Can you work these out from the drawing? Everything is in mm from the part's minimum corner. Coordinates: 2 decimals unless noted, no trailing zeros. Order: outer loops, then holes, each group sorted by start corner. A loop starts at its lowest first (then second) coordinate and runs counter-clockwise, first axis right, second up. Notation, with made-up numbers: (43, -31) -> (101, -31) arc R16 cw to (101, -5) -> close; hole circle Ø3 at (63.25, 82.5). An arc over 180 degrees is marked (long way). Return JSON: item names as keys, results as strings. Group by question number.
1) If I drill on probe 1 along Y at (x, z) = (93, 0.85); probe 2 along Y at (x, z) = (5, 0.9); probe 3 along X at (y, z) = (60, 1.85), over which ranges is the centre line in solid material (lowest first)? Write a range as from..to.
2) If we section it at B-B, the plane x = 35: Please give me the cut outline in (y, z), then the cut area to 3 significant figures.
3) For pin 1 (1.5 mm diameter, centred on x = 93, y = 59, fed in from +Z), with a flat end and sliding along its axis, tell me the tip position at first contact or that it passes through.
4) If we section it at A-A, the plane y = 10: Please give me the cut outline in (x, z), then the cut area to 3 significant figures.
5) If we section it at C-C, the plane x = 5: Please give me the cut outline in (y, z), then the cut area to 3 significant figures.
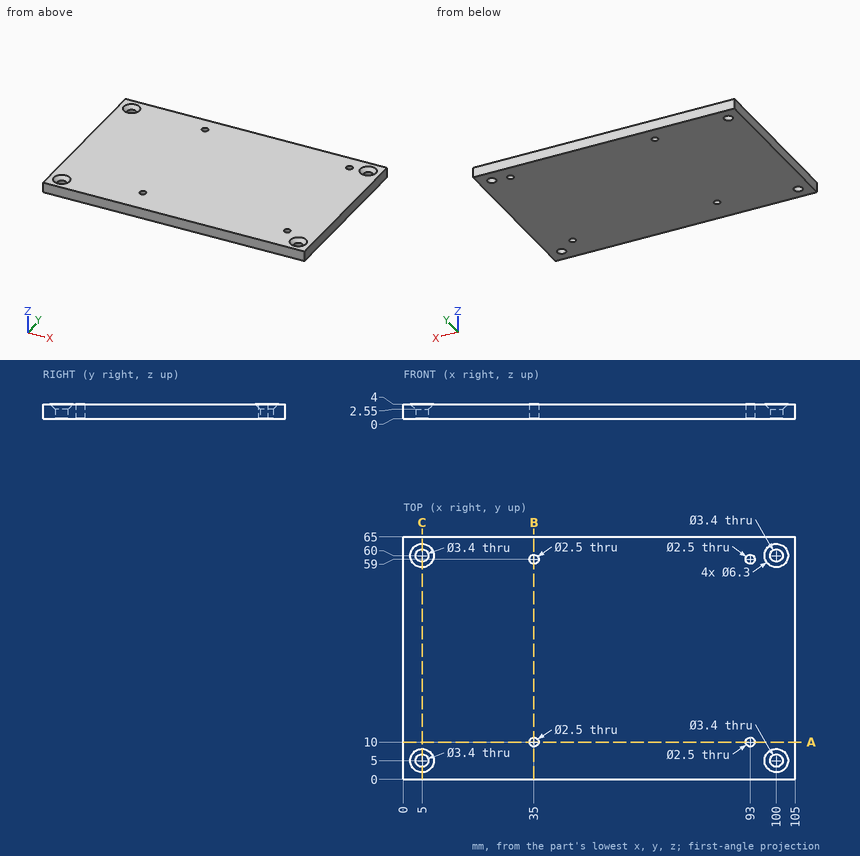
Result sheet:
{
 "1": {"probe 1": "y = 0..8.75, 11.25..57.75, 60.25..65", "probe 2": "y = 0..3.3, 6.7..58.3, 61.7..65", "probe 3": "x = 0..3.3, 6.7..34.25, 35.75..92.25, 93.75..98.3, 101.7..105"},
 "2": {"outline": "(0, 0) -> (8.75, 0) -> (8.75, 4) -> (0, 4) -> close; (11.25, 0) -> (57.75, 0) -> (57.75, 4) -> (11.25, 4) -> close; (60.25, 0) -> (65, 0) -> (65, 4) -> (60.25, 4) -> close", "area": "240 mm2"},
 "3": {"pin 1": "passes through"},
 "4": {"outline": "(0, 0) -> (33.75, 0) -> (33.75, 4) -> (0, 4) -> close; (36.25, 0) -> (91.75, 0) -> (91.75, 4) -> (36.25, 4) -> close; (94.25, 0) -> (105, 0) -> (105, 4) -> (94.25, 4) -> close", "area": "400 mm2"},
 "5": {"outline": "(0, 0) -> (3.3, 0) -> (3.3, 2.55) -> (1.85, 4) -> (0, 4) -> close; (6.7, 0) -> (58.3, 0) -> (58.3, 2.55) -> (56.85, 4) -> (8.15, 4) -> (6.7, 2.55) -> close; (61.7, 0) -> (65, 0) -> (65, 4) -> (63.15, 4) -> (61.7, 2.55) -> close", "area": "229 mm2"}
}
